```python
from build123d import *

# Parameters (mm, degrees)
BOSS_EXTRUDE1_DEPTH                                  = 7
M3_CLEARANCE_HOLE1_D                                 = 3.6
CUT_EXTRUDE1_DEPTH                                   = 22.16158075380949
CUT_EXTRUDE1_DEPTH_BACK                              = 2
BOSS_EXTRUDE2_DEPTH                                  = 5
FILLET1_R                                            = 5.5
CHAMFER1_SIZE                                        = 1
CBORE_FOR_M3_HEXAGON_SOCKET_HEAD_CAP_SCR_D           = 3.6
CBORE_FOR_M3_HEXAGON_SOCKET_HEAD_CAP_SCR_CBORE_D     = 6
CBORE_FOR_M3_HEXAGON_SOCKET_HEAD_CAP_SCR_CBORE_DEPTH = 4.4
FILLET2_R                                            = 2


with BuildPart() as part:
    # Sketch1 → Boss-Extrude1 (new body)
    with BuildSketch(Plane(origin=(0, 0, 0), x_dir=(1, 0, 0), z_dir=(0, 1, 0))):
        Polygon((16.5, -11.249999999999996), (-16.499999999999996, -11.250000000000002), (-16.499999999999996, 11.249999999999998), (16.500000000000004, 11.250000000000002), align=None)
    extrude(amount=BOSS_EXTRUDE1_DEPTH)

    # M3 Clearance Hole1 (through all)
    with Locations(Plane(origin=(-14, 7, -6.25), x_dir=(0, 0, 1), z_dir=(0, 1, 0))):
        with Locations((0, 0), (0, 28), (15, 28), (15, 0)):
            Hole(M3_CLEARANCE_HOLE1_D / 2)

    # Sketch7 → Cut-Extrude1 (cut, two sides: drawn at the far end of the back side and taken through both)
    with BuildSketch(Plane.XZ.offset(-CUT_EXTRUDE1_DEPTH_BACK)):
        Polygon((-1.78e-15, 7.784737974375178), (-14.605868156846089, -11.250000000000002), (14.605868156846089, -11.250000000000002), align=None)
    extrude(amount=CUT_EXTRUDE1_DEPTH + CUT_EXTRUDE1_DEPTH_BACK, mode=Mode.SUBTRACT)

    # Sketch8 → Boss-Extrude2 (add)
    with BuildSketch(Plane.XZ.offset(-2)):
        Polygon((-16.499999999999996, -11.249999999999998), (16.500000000000004, -11.250000000000002), (16.500000000000004, -18.749999999999996), (-16.499999999999996, -18.749999999999996), align=None)
    extrude(amount=-BOSS_EXTRUDE2_DEPTH)

    # Fillet1
    fillet1_edges = [part.edges().sort_by_distance(p)[0] for p in [
        (0, 1, 7.784737974375178),
    ]]
    fillet(fillet1_edges, radius=FILLET1_R)

    # Chamfer1
    chamfer1_edges = [part.edges().sort_by_distance(p)[0] for p in [
        (16.500000000000004, 4.5, -18.749999999999996),
        (-16.499999999999996, 4.5, -18.749999999999996),
        (16.5, 3.5, 11.249999999999996),
        (-16.499999999999996, 3.5, 11.250000000000002),
    ]]
    chamfer(chamfer1_edges, length=CHAMFER1_SIZE)

    # CBORE for M3 Hexagon socket head cap screws1 (through all)
    with Locations(Plane(origin=(-8, 0, 0.5), x_dir=(0, 0, -1), z_dir=(0, -1, 0))):
        with Locations((0, 0), (0, 16), (16, 0), (16, 16)):
            CounterBoreHole(CBORE_FOR_M3_HEXAGON_SOCKET_HEAD_CAP_SCR_D / 2, CBORE_FOR_M3_HEXAGON_SOCKET_HEAD_CAP_SCR_CBORE_D / 2, CBORE_FOR_M3_HEXAGON_SOCKET_HEAD_CAP_SCR_CBORE_DEPTH)

    # Fillet2
    # the kernel refuses this fillet: 2 mm, written as the material it takes off along each edge
    with BuildSketch(Plane(origin=(7.890215098826709, 2, -2.497990539590539), x_dir=(0.6087614290087221, 0, -0.793353340291234), z_dir=(0, -1, 0))) as fillet2_piece_1:
        with BuildLine():
            CenterArc((2.6875953448217693, 1.9999999999999998), FILLET2_R, 181.00663294290118, 88.9933670570988)
            ThreePointArc((0.6879040087236102, 1.9648636892380578), (0.5198514245240395, 0.9208489893174272), (0, 0))
            Line((0, 0), (2.687595344821769, -6e-17))
        make_face()
    extrude(amount=8.718988362054422, mode=Mode.SUBTRACT)
    with BuildSketch(Plane(origin=(5.075749087550851, 2, 1.169892977303331), x_dir=(0.5345809158392569, 0, 0.8451172962497344), z_dir=(0, -1, 0))) as fillet2_piece_2:
        with BuildLine():
            CenterArc((2.658961571108191, 1.8862980173372965), FILLET2_R, 171.49145576395077, 79.09584417917802)
            Line((0.6809739505501902, 2.182211810390776), (0.48317518849439006, 2.2118031896961234))
            ThreePointArc((0.48317518849439006, 2.2118031896961234), (0.21601574537907067, 1.167239486619447), (-0.18771727363639942, 0.06900887753410519))
            Line((-0.18771727363639942, 0.06900887753410519), (0.06647403927770486, -0.18862980173372967))
            ThreePointArc((0.06647403927770486, -0.18862980173372967), (0.9971105891655724, -0.02944702600594452), (1.9277471390534389, -0.18862980173372967))
            Line((1.9277471390534389, -0.18862980173372967), (1.9942211783311437, -1.1e-16))
        make_face()
    extrude(amount=7.714987919244077, mode=Mode.SUBTRACT)
    with BuildSketch(Plane(origin=(-5.075749087550852, 2, 1.169892977303333), x_dir=(0.6475032352688438, 0, 0.76206270104), z_dir=(0, -1, 0))) as fillet2_piece_3:
        with BuildLine():
            CenterArc((2.5927374915549515, 1.9763373059158453), FILLET2_R, 182.08181462888786, 79.09584417902704)
            Line((0.594057543639052, 1.9036842550583746), (0.39418954884746193, 1.8964189499726276))
            ThreePointArc((0.39418954884746193, 1.8964189499726276), (0.2689186301864014, 0.960614087293723), (-0.16026415854934645, 0.11964697858479319))
            Line((-0.16026415854934645, 0.11964697858479319), (0.00995689513411226, -0.19975199683429518))
            ThreePointArc((0.00995689513411226, -0.19975199683429518), (1.1785960560365805, -0.14149967515975187), (2.2553209353120622, -0.19763373059158465))
            Line((2.2553209353120622, -0.19763373059158465), (2.2859951676977794, 3e-17))
        make_face()
    extrude(amount=7.714987919244448, mode=Mode.SUBTRACT)
    with BuildSketch(Plane(origin=(-7.890215098826712, 2, -2.497990539590539), x_dir=(-0.9499463523512466, 0, 0.3124130721569783), z_dir=(0, -1, 0))) as fillet2_piece_4:
        with BuildLine():
            CenterArc((2.7757365364902538, 1.8757546261437203), FILLET2_R, 160.70471375400504, 88.99336705710107)
            Line((0.8880802565250356, 2.53662811532896), (0, 0))
            ThreePointArc((0, 0), (1.040901201183847, 0.18636806078441912), (2.0818024023676904, -4e-17))
        make_face()
    extrude(amount=8.718988362054088, mode=Mode.SUBTRACT)


solid = part.part
```
Input: part model. Units: mm. Frame: model coordinates. A direction names the side the tool comes from. Give positions to 0.01 mm unless a question says otherwise; leave off trailing zeros. Order: outer loops, then holes, each group sorted by start corner. A loop starts at its lowest first (then second) coordinate and runs counter-clockwise, first axis right, second up. Notation, with made-up numbers: (-15, 23) - (0, 23) arc R6 ccw to (0, 33) - close; hole circle Ø9 at (-15.75, -19.5). An arc over 180 degrees is marked (long way). One line per item, written item: value.
1. Cut plane D-D, the plane z = 8.75. Output: boundary loops of the cut face in (x, y), and give its area (3 significant figures).
Determined:
outline: (-16.5, 0) - (-15.8, 0) - (-15.8, 7) - (-16.5, 7) - close; (-12.2, 0) - (12.2, 0) - (12.2, 7) - (-12.2, 7) - close; (15.8, 0) - (16.5, 0) - (16.5, 7) - (15.8, 7) - close
area: 181 mm2
2. Pin query (flat end, axial travel): pin 1 Ø9.5 at (x, z) = (-8, -15.5) entering from -Y; pin 2 Ø1.5 at (x, y) = (15, 1) entering from -Z; pin 3 Ø2 at (x, y) = (-16, 0.5) entering from -Z. Return the tip coordinate at first contact, or that it passes through.
Determined:
pin 1: y = 2
pin 2: z = -11.25
pin 3: z = -11.25
3. Draft query along Z for faces 6 (the face through (15.99, 3.45, 10.76)), 7 (the face through (15.217, 3.451, 10.077)), 8 (the face through (16.5, 3, -4)). Return one class per face: released by +Z, released by -Z, zero draft, split by the parting line, or undercut.
Determined:
face 6: released by +Z
face 7: undercut
face 8: zero draft
4. Cut plane B-B, the plane y = 2.5. Give the number of separate pieces and of enclosed holes in the cut face, and give its area (3 significant figures).
Determined:
separate pieces: 1
enclosed holes: 8
area: 834 mm2
5. Cut plane C-C, the plane x = 8. Output: boundary loops of the cut face in (y, z), and give its area (3 significant figures).
Determined:
outline: (0, 3.5) - (4.4, 3.5) - (4.4, 2.3) - (7, 2.3) - (7, 11.25) - (0, 11.25) - close; (2, -18.75) - (7, -18.75) - (7, -17.3) - (4.4, -17.3) - (4.4, -18.5) - (2, -18.5) - close; (2, -12.5) - (4.4, -12.5) - (4.4, -13.7) - (7, -13.7) - (7, -1.3) - (4.4, -1.3) - (4.4, -2.5) - (2, -2.5) - close
area: 118 mm2
6. Cut plane A-A, the plane z = 0.5. Output: boundary loops of the cut face in (x, y), and give its area (3 significant figures).
Determined:
outline: (-16.5, 0) - (-11, 0) - (-11, 4.4) - (-9.8, 4.4) - (-9.8, 7) - (-16.5, 7) - close; (-6.2, 4.4) - (-5, 4.4) - (-5, 2) - (5, 2) - (5, 4.4) - (6.2, 4.4) - (6.2, 7) - (-6.2, 7) - close; (9.8, 4.4) - (11, 4.4) - (11, 0) - (16.5, 0) - (16.5, 7) - (9.8, 7) - close
area: 139 mm2
7. Line query: probe 1 along X at (y, z) = (3.1, 0.5); probe 2 along X at (y, z) = (5.5, 0.5); probe 3 along Z at (x, y) = (-8.5, 4.75). Output: solid intervals per line, ascending.
Determined:
probe 1: -16.5 to -11, -5 to 5, 11 to 16.5
probe 2: -16.5 to -9.8, -6.2 to 6.2, 9.8 to 16.5
probe 3: -18.75 to -17.23, -13.77 to -1.23, 2.23 to 11.25
8. Reachability of faces 1 (the face through (-16, 1, -11.25)), 2 (the face through (-0.05, 0.99, 4.25)), 3 (the face through (0, 7, -4)), 4 (the face through (0, 4, -18.75)), 5 (the face through (-10, 4.4, 1)) from +Z, -Z, +X, -X, +Y, -Y: full face, straight path, thin tool, end or side. Return the list, or none.
Determined:
face 1: -Z, +X, -X, -Y
face 2: -Z, -Y
face 3: +Z, -Z, +X, -X, +Y
face 4: -Z, +X, -X, +Y, -Y
face 5: -Y
